from build123d import *

# Parameters (mm, degrees)
EXTRUDE_1_DEPTH     = 3
SKETCH_2_R          = 1.575
SKETCH_2_R_2        = 1.6
CUT_EXTRUDE_1_DEPTH = 91.321647461


with BuildPart() as part:
    # 草图1 → 凸台-拉伸1 (new body)
    with BuildSketch(Plane.XY):
        Polygon((0, 0), (22, 0), (57, 0), (57, -15), (57, -55), (22, -70), (0, -70), (-40, -70), (-40, -55), (-40, -15), align=None)
    extrude(amount=EXTRUDE_1_DEPTH)

    # 草图2 → 切除-拉伸1 (cut, through all)
    with BuildSketch(Plane.XY.offset(3)):
        with Locations((18.5, -5)):
            Circle(SKETCH_2_R)
        with Locations(Location((18.5, -15, 0), (0, 0, 180))):
            Circle(SKETCH_2_R)
        with Locations((3.5, -15)):
            Circle(SKETCH_2_R)
        with Locations(Location((3.5, -5, 0), (0, 0, 180))):
            Circle(SKETCH_2_R)
        with Locations((3.5, -65)):
            Circle(SKETCH_2_R)
        with Locations(Location((3.5, -55, 0), (0, 0, 180))):
            Circle(SKETCH_2_R)
        with Locations((18.5, -55)):
            Circle(SKETCH_2_R)
        with Locations(Location((18.5, -65, 0), (0, 0, 180))):
            Circle(SKETCH_2_R)
        with Locations((-19, -42.5)):
            Circle(SKETCH_2_R)
        with Locations(Location((-19, -27.5, 0), (0, 0, 180))):
            Circle(SKETCH_2_R)
        with Locations(Location((-9, -42.5, 0), (0, 0, 180))):
            Circle(SKETCH_2_R)
        with Locations((-9, -27.5)):
            Circle(SKETCH_2_R)
        with Locations((31, -42.5)):
            Circle(SKETCH_2_R)
        with Locations(Location((41, -42.5, 0), (0, 0, 180))):
            Circle(SKETCH_2_R)
        with Locations((41, -27.5)):
            Circle(SKETCH_2_R)
        with Locations(Location((31, -27.5, 0), (0, 0, 180))):
            Circle(SKETCH_2_R)
        with Locations((-35, -65)):
            Circle(SKETCH_2_R_2)
        with Locations(Location((-25, -65, 0), (0, 0, 180))):
            Circle(SKETCH_2_R_2)
        with Locations((-25, -55)):
            Circle(SKETCH_2_R_2)
        with Locations(Location((-35, -55, 0), (0, 0, 180))):
            Circle(SKETCH_2_R_2)
        with Locations((-5, -55)):
            Circle(SKETCH_2_R_2)
        with Locations(Location((-15, -55, 0), (0, 0, 180))):
            Circle(SKETCH_2_R_2)
        with Locations((-15, -65)):
            Circle(SKETCH_2_R_2)
        with Locations(Location((-5, -65, 0), (0, 0, 180))):
            Circle(SKETCH_2_R_2)
        with Locations((52, 1)):
            Circle(SKETCH_2_R_2)
        with Locations((42, 1)):
            Circle(SKETCH_2_R_2)
        with Locations(Location((52, -9, 0), (0, 0, 180))):
            Circle(SKETCH_2_R_2)
        with Locations((42, -9)):
            Circle(SKETCH_2_R_2)
        Polygon((3.5, -30.5), (3.5, -42.5), (12.5, -42.5), align=None)
        Polygon((9.5, -27.5), (18.5, -39.5), (18.5, -27.5), align=None)
    extrude(amount=-CUT_EXTRUDE_1_DEPTH, mode=Mode.SUBTRACT)


solid = part.part
Source: CAD feature listing. Evaluate the final solid. Frame: model axes, mm. A direction names the side the tool comes from. Round coordinates to 2 decimals unless told otherwise and drop trailing zeros. Loops run counter-clockwise (first coordinate to the right, second up) from the corner with the lowest first, then second, coordinate; pieces in that order, holes last. Notation, with made-up numbers: (-2, 79) - (10, 79) arc R13 cw to (10, 97) - close; hole circle Ø7 at (27, 88). An arc over 180 degrees is marked (long way). Write item = value, one per line. Start each with the question number.
Item 1: Material intervals for line 1 (Y direction, x = -15, z = 2) (3 decimals); line 2 (Y direction, x = 11, z = 0.9); line 3 (X direction, y = -43, z = 2.3), sorted ascending.
Item 2: First-contact query: pin 1 Ø2.5 at (x, y) = (41, -42.5) entering from -Z; pin 2 Ø1 at (x, z) = (38, 0.5) entering from -Y. Flat tips, straight axial feed; report the tip coordinate or a pass-through.
Item 3: Section query A-A on y = -9. Output: boundary loops of the cut face in (x, z), plus the area to 3 significant figures.
Item 4: Section query C-C on x = 52. Output: boundary loops of the cut face in (y, z).
Item 5: Reachability of faces 1 (the face through (8, -42.5, 2)), 2 (the face through (-20.28, -7.605, 1.479)) from +Z, -Z, +X, -X, +Y, -Y: full face, straight path, thin tool, end or side. Return the list, or none.
Item 6: Section query B-B on x = -5. Output: boundary loops of the cut face in (y, z) (3 decimals), plus the area to 3 significant figures.
Item 7: Section query D-D on z = 1.2. Count the separate pieces of the cut face and the enclosed holes in it, plus the area to 3 significant figures.
Results list:
q1.line_1 = -70 to -66.6, -63.4 to -56.6, -53.4 to -5.625
q1.line_2 = -70 to -42.5, -40.5 to -29.5, -27.5 to 0
q1.line_3 = -40 to -20.49, -17.51 to -10.49, -7.51 to 29.51, 32.49 to 39.51, 42.49 to 57
q2.pin_1 = through
q2.pin_2 = -63.36
q3.outline = (-24, 0) - (40.4, 0) - (40.4, 3) - (-24, 3) - close; (43.6, 0) - (50.4, 0) - (50.4, 3) - (43.6, 3) - close; (53.6, 0) - (57, 0) - (57, 3) - (53.6, 3) - close
q3.area = 224 mm²
q4.outline = (-57.14, 0) - (-10.6, 0) - (-10.6, 3) - (-57.14, 3) - close; (-7.4, 0) - (-0.6, 0) - (-0.6, 3) - (-7.4, 3) - close
q5.face_1 = +Z, -Z
q5.face_2 = +Z, -Z, -X, +Y
q6.outline = (-70, 0) - (-66.6, 0) - (-66.6, 3) - (-70, 3) - close; (-63.4, 0) - (-56.6, 0) - (-56.6, 3) - (-63.4, 3) - close; (-53.4, 0) - (-1.875, 0) - (-1.875, 3) - (-53.4, 3) - close
q6.area = 185 mm²
q7.separate_pieces = 1
q7.enclosed_holes = 28
q7.area = 5,910 mm²
